Can you work these out from the model? Positions are in its coordinate system, mm. A direction names the side the tool comes from. Give positions to 0.01 mm unless a question says otherwise; leave off trailing zeros. Loops run counter-clockwise (first coordinate to the right, second up) from the corner with the lowest first, then second, coordinate; pieces in that order, holes last. Notation, with made-up numbers: (-37.5, 32.5) -> (-1.5, 32.5) arc R26 ccw to (-1.5, 68.5) -> close; hole circle Ø9 at (25, -20). An arc over 180 degrees is marked (long way). Use CSV: the item, a comma, the result in double quotes.
from build123d import *

# Parameters (mm, degrees)
ESQUISSE1_ONE_SIDE_W         = 80
ESQUISSE1_ONE_SIDE_H         = 30
ESQUISSE1_ONE_SIDE_W_2       = 100
ESQUISSE1_ONE_SIDE_H_2       = 630
ENL_V_MAT_EXTRU_2_DEPTH      = 952.933780363
ENL_V_MAT_EXTRU_2_DEPTH_BACK = 952.933780363
ESQUISSE2_R                  = 25


with BuildPart() as part:
    # Esquisse1 one side → Révolution1 (revolve)
    with BuildSketch(Plane.XY, mode=Mode.PRIVATE) as r_volution1_sk:
        with BuildLine():
            Line((0, 552.370333546), (0, 602.370333546))
            ThreePointArc((0, 602.370333546), (-25, 577.370333546), (0, 552.370333546))
        make_face()
        with BuildLine():
            Line((0, 693.136902569), (100, 693.136902569))
            ThreePointArc((100, 693.136902569), (129.068087767, 845.351432312), (0, 931.11649228))
            Line((0, 931.11649228), (0, 693.136902569))
        make_face()
        with BuildLine():
            ThreePointArc((100, 693.136902569), (82.774757951, 660.253618058), (100, 627.370333546))
            Line((100, 627.370333546), (0, 627.370333546))
            Line((0, 627.370333546), (0, 693.136902569))
            Line((0, 693.136902569), (100, 693.136902569))
        make_face()
        Polygon((0, 527.370333546), (0, 627.370333546), (100, 627.370333546), (100, 527.370333546), (80, 527.370333546), align=None)
        with Locations((40, 512.370333546)):
            Rectangle(ESQUISSE1_ONE_SIDE_W, ESQUISSE1_ONE_SIDE_H)
        with BuildLine():
            ThreePointArc((0, 602.370333546), (-25, 577.370333546), (0, 552.370333546))
            Line((0, 552.370333546), (0, 602.370333546))
        make_face()
        with BuildLine():
            Line((0, 602.370333546), (0, 552.370333546))
            ThreePointArc((0, 552.370333546), (17.67766953, 559.692664016), (25, 577.370333546))
            ThreePointArc((25, 577.370333546), (17.67766953, 595.048003076), (0, 602.370333546))
        make_face()
        with Locations((50, 182.370333546)):
            Rectangle(ESQUISSE1_ONE_SIDE_W_2, ESQUISSE1_ONE_SIDE_H_2)
        Polygon((100, -132.629666454), (0, -132.629666454), (0, -152.629666454), (80, -152.629666454), align=None)
    revolve(r_volution1_sk.sketch.rotate(Axis((0, -208.828974679, 0), (0, 1, 0)), 90), axis=Axis((0, -208.828974679, 0), (0, 1, 0)))

    # Esquisse2 → Enlèv. mat.-Extru.2 (cut, two sides: drawn at the far end of the back side and taken through both)
    with BuildSketch(Plane.XY.offset(-ENL_V_MAT_EXTRU_2_DEPTH_BACK)):
        with Locations((0, 577.370333546)):
            Circle(ESQUISSE2_R)
    extrude(amount=ENL_V_MAT_EXTRU_2_DEPTH + ENL_V_MAT_EXTRU_2_DEPTH_BACK, mode=Mode.SUBTRACT)


solid = part.part
(1) If I drill on L1, parallel to Y at x = 23, z = 87.5; L2, parallel to Y at x = 0, z = 7; L3, parallel to X at y = -48.5, z = -3, over which ranges is the centre line in solid material (lowest first)? Write a range as from..to.
Answer sheet:
L1,"y = -142.16..497.37, 527.37..567.57, 587.17..636.66, 683.85..897.96"
L2,"y = -152.63..552.37, 602.37..930.94"
L3,"x = -99.95..99.95"
(2) If we section it at A-A, the plane x = 0: Write out the boundary of the cut face in (y, z), then the cut area to 3 significant figures.
Answer sheet:
outline,"(-152.63, -80) -> (-132.63, -100) -> (497.37, -100) -> (497.37, -80) -> (527.37, -80) -> (527.37, -100) -> (552.37, -100) -> (552.37, 100) -> (527.37, 100) -> (527.37, 80) -> (497.37, 80) -> (497.37, 100) -> (-132.63, 100) -> (-152.63, 80) -> close; (602.37, -100) -> (627.37, -100) arc R40 cw to (693.14, -100) arc R140 ccw (long way) to (693.14, 100) arc R40 cw to (627.37, 100) -> (602.37, 100) -> close"
area,"212,000 mm2"
(3) We'd pull the mould along Y, two halves only. Please class faces 3 (the face through (-3.25, 602.16, -1.4)), 4 (the face through (-1, -152.63, -1)), 5 (the face through (-30.04, 186.78, -95.38)): released by +Y, released by -Y, zero draft, split by the parting line, or undercut.
Answer sheet:
face 3,"undercut"
face 4,"released by -Y"
face 5,"zero draft"
(4) Which directions (+Z, -Z, +X, -X, +Y, -Y) give clear straight access to the entire face, cutting with the end or side of a thin tool? Please do faces 1 (the face through (-3.517, 512.58, 79.923)), 2 (the face through (-30.04, 576.67, -95.38)).
Answer sheet:
face 1,"none"
face 2,"-Y"
(5) If we section it at D-D, the plane z = -116: Write out the boundary of the cut face in (x, y).
Answer sheet:
outline,"circle Ø156.77 at (0, 791.12)"
(6) If we section it at B-B, the plane z = 0: Write out the boundary of the cut face in (x, y), then the cut area to 3 significant figures.
Answer sheet:
outline,"(-100, -132.63) -> (-80, -152.63) -> (80, -152.63) -> (100, -132.63) -> (100, 497.37) -> (80, 497.37) -> (80, 527.37) -> (100, 527.37) -> (100, 627.37) arc R40 cw to (100, 693.14) arc R140 ccw (long way) to (-100, 693.14) arc R40 cw to (-100, 627.37) -> (-100, 527.37) -> (-80, 527.37) -> (-80, 497.37) -> (-100, 497.37) -> close; hole circle Ø50 at (0, 577.37)"
area,"220,000 mm2"
(7) If we section it at C-C, the plane y = 134.5: Write out the boundary of the cut face in (x, z), then the cut area to 3 significant figures.
Answer sheet:
outline,"circle Ø200 at (0, 0)"
area,"31,400 mm2"
(8) Will these pins go through, and if not, where does the flat tip stop? pin 1 Ø3 at (x, z) = (36, -8) entering from +Y; pin 2 Ø1 at (x, y) = (-29, 134) entering from -Z; pin 3 Ø8 at (x, z) = (-105, -43.5) entering from +Y.
Answer sheet:
pin 1,"stops at y = 926.57"
pin 2,"stops at z = -95.85"
pin 3,"stops at y = 878.16"
